Check sheet for the modelled part. Datum: model origin and axes. Units: mm. Face numbers are marked on the shaded views. A direction names the side the tool comes from. Round coordinates to 2 decimals unless told otherwise and drop trailing zeros. Write each loop counter-clockwise with the first axis right and the second up, starting at its lowest first coordinate (ties: lowest second). Pieces come first, ordered by that corner, then holes. Notation, with made-up numbers: (84.25, 71.5) -> (109.25, 71.5) arc R25 cw to (109.25, 90.5) -> close; hole circle Ø9 at (77, 63). An arc over 180 degrees is marked (long way). Put each result on its own line as item: value. Start each with the question number.
from build123d import *

# Parameters (mm, degrees)
SKETCH_1_R          = 1.65
EXTRUDE_1_DEPTH     = 3
EXTRUDE_2_DEPTH     = 3
CUT_EXTRUDE_1_REACH = 30.673
SKETCH_3_R          = 0.75


with BuildPart() as part:
    # 草图1 → 凸台-拉伸1 (new body)
    with BuildSketch(Plane(origin=(0, 0, 0), x_dir=(1, 0, 0), z_dir=(0, 1, 0))):
        with BuildLine():
            Line((0, 3), (23.05, 3))
            ThreePointArc((23.05, 3), (26.05, 0), (23.05, -3))
            Line((23.05, -3), (0, -3))
            ThreePointArc((0, -3), (-3, 0), (0, 3))
        make_face()
        with Locations(Location((23.05, 0, 0), (0, 0, 270))):
            Circle(SKETCH_1_R, mode=Mode.SUBTRACT)
    extrude(amount=EXTRUDE_1_DEPTH)

    # 草图2 → 凸台-拉伸2 (add)
    with BuildSketch(Plane(origin=(0, 0, 0), x_dir=(1, 0, 0), z_dir=(0, 1, 0))):
        with BuildLine():
            Line((3, 0), (3, -8.6))
            ThreePointArc((3, -8.6), (0, -11.6), (-3, -8.6))
            Line((-3, -8.6), (-3, 0))
            ThreePointArc((-3, 0), (0, 3), (3, 0))
        make_face()
    extrude(amount=EXTRUDE_2_DEPTH)

    # 草图3 → 切除-拉伸1 (cut, up to next)
    with BuildSketch(Plane(origin=(0, 3, 0), x_dir=(1, 0, 0), z_dir=(0, 1, 0)), mode=Mode.PRIVATE) as cut_extrude_1_sk1:
        with Locations(Location((0, -8.6, 0), (0, 0, 270))):
            Circle(SKETCH_3_R)
    cut_extrude_1_tool1 = extrude(cut_extrude_1_sk1.sketch, amount=-CUT_EXTRUDE_1_REACH, mode=Mode.PRIVATE) & part.part
    add(cut_extrude_1_tool1.solids().sort_by_distance((0, 3, 8.6))[0], mode=Mode.SUBTRACT)


solid = part.part
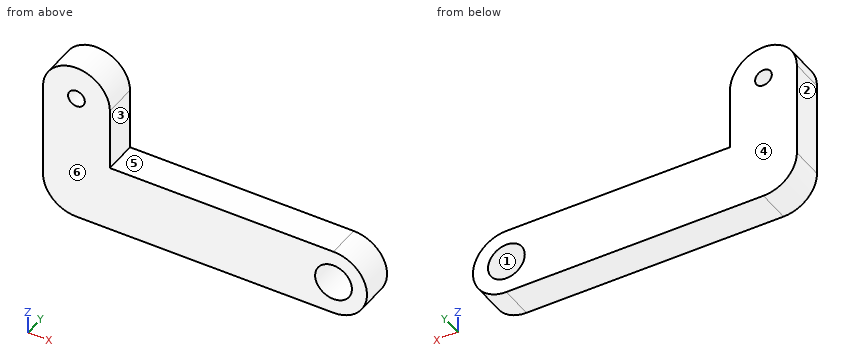
1. Material ranges on L1, parallel to X at y = 2.3, z = 0; L2, parallel to X at y = 1.75, z = 8.6; L3, parallel to Z at x = 10.5, y = 0.45, recorded low to high. Write a range as [from, to].
2. Section check B-B, the plane z = -1. Enter the section's corners in (x, y), then the cut area to 3 significant figures.
3. Gauge pin test, flat ends, axial feed: P1, Ø2, axis at x = 23.05, z = 0, coming from the +Y side; P2, Ø1.5, axis at x = 10.5, y = 2, coming from the +Z side. Record the tip position at first contact, or that the pin passes through.
4. Section check C-C, the plane x = 24. Enter the section's corners in (y, z).
5. Section check D-D, the plane x = 14.5. Enter the section's corners in (y, z), then the cut area to 3 significant figures.
6. Draft check along X on the marked faces 1, 2, 3 and 4. Enter one of: released by +X, released by -X, zero draft, split by the parting line, or undercut.
7. Access from +Z, -Z, +X, -X, +Y, -Y to the whole of each face (thin tool, end or side, straight path). Record for the marked faces 5 and 6.
8. Section check A-A, the plane y = 2.4. Enter the section's corners in (x, z).
Reply:
1. L1: x = [-3, 21.4], [24.7, 26.05]
1. L2: x = [-3, -0.75], [0.75, 3]
1. L3: z = [-3, 3]
2. outline: (-2.83, 0) -> (21.74, 0) -> (21.74, 3) -> (-2.83, 3) -> close; (24.36, 0) -> (25.88, 0) -> (25.88, 3) -> (24.36, 3) -> close
2. area: 78.2 mm2
3. P1: passes through
3. P2: stops at z = 3
4. outline: (0, -2.85) -> (3, -2.85) -> (3, -1.35) -> (0, -1.35) -> close; (0, 1.35) -> (3, 1.35) -> (3, 2.85) -> (0, 2.85) -> close
5. outline: (0, -3) -> (3, -3) -> (3, 3) -> (0, 3) -> close
5. area: 18.0 mm2
6. face 1: undercut
6. face 2: released by -X
6. face 3: released by +X
6. face 4: zero draft
7. face 5: +Z, +X, +Y, -Y
7. face 6: +Z, -Z, +X, -X, -Y
8. outline: (-3, 0) arc R3 ccw to (0, -3) -> (23.05, -3) arc R3 ccw to (23.05, 3) -> (3, 3) -> (3, 8.6) arc R3 ccw to (-3, 8.6) -> close; hole circle Ø1.5 at (0, 8.6); hole circle Ø3.3 at (23.05, 0)
